Read the model definition and answer for the solid it produces. Units are mm, in the model's axes. A direction names the side the tool comes from. Coordinates: 2 decimals unless noted, no trailing zeros. Order: outer loops, then holes, each group sorted by start corner. A loop starts at its lowest first (then second) coordinate and runs counter-clockwise, first axis right, second up. Notation, with made-up numbers: (14, 23) -> (42, 23) arc R10 cw to (42, 32) -> close; hole circle Ø8 at (2, -0.5). An arc over 180 degrees is marked (long way). Answer as a JSON object with one key per item and string values. Group by question number.
1) Section D-D on z = 5.25 is taken. Determine the outline of the cut face in (x, y), and give its area (3 significant figures).
2) Section B-B on x = 86 is taken. Determine the outline of the cut face in (y, z), and give its area (3 significant figures).
3) Determine the mould class of faces 4 (the flat face through (13, 0, 0)), 5 (the cylindrical face through (128.719, -5.594, 10.26)), 6 (the cylindrical face through (119, 0, 10)), 7 (the cylindrical face through (4.8, -2.4, 0.7)) for opening direction X: released by +X, released by -X, zero draft, split by the parting line, or undercut.
4) Consider L1, parallel to Y at x = 8, z = 0.75; L2, parallel to Z at x = 15.5, y = 0.75; L3, parallel to Z at x = 49, y = -1.5. Determine where each line is inside the solid, lowest interval first.
5) A tool of negligible diameter and unlimited length cuts with its end or side. For faces 1 (the flat face through (82, 0, 9.5)), 2 (the flat face through (66, 8, 10)), 3 (the flat face through (13, 0, 1.5)), from which of +Z, -Z, +X, -X, +Y, -Y can it reach the whole face along a straight path? Write none if from no direction.
6) Given pin 1 (8 mm diameter, centred on x = 11.5, y = -0.5, fed in from +Z); pin 2 (5 mm diameter, centred on y = 2, z = 3, fed in from +X), each flat-ended and moving along its own axis, determine where each tip first touches the part or whether it passes through.
7) Section A-A on y = -1.25 is taken. Determine the outline of the cut face in (x, z).
8) Section C-C on y = -6.5 is taken. Determine the outline of the cut face in (x, z), and give its area (3 significant figures).
from build123d import *

# Parameters (mm, degrees)
EXTRUDE_1_DEPTH          = 8
FILLET_1_R               = 8
CUT_EXTRUDE_1_DEPTH      = 132.587423411
CUT_EXTRUDE_1_DEPTH_BACK = 132.587423411
SKETCH_2_R               = 4


with BuildPart() as part:
    # 草图1 → 拉伸-薄壁1 (new, symmetric)
    with BuildSketch(Plane(origin=(0, 0, 0), x_dir=(1, 0, 0), z_dir=(0, 1, 0))):
        Polygon((0, 0), (18, 0), (34, -9.5), (131, -9.5), (131, -11), (33.588243042, -11), (17.588243042, -1.5), (0, -1.5), align=None)
    extrude(amount=EXTRUDE_1_DEPTH, both=True)

    # 圆角1
    fillet_1_edges = [part.edges().sort_by_distance(p)[0] for p in [
        (131, -8, 10.25),
        (131, 8, 10.25),
        (0, -8, 0.75),
        (0, 8, 0.75),
    ]]
    fillet(fillet_1_edges, radius=FILLET_1_R - 0.0001)  # a hair under: the kernel refuses the full size

    # 草图2 → 切除-拉伸1 (cut, two sides: drawn at the far end of the back side and taken through both)
    with BuildSketch(Plane.XY.offset(1.5).offset(-CUT_EXTRUDE_1_DEPTH_BACK)):
        with Locations((8, 0)):
            Circle(SKETCH_2_R)
        with Locations((123, 0)):
            Circle(SKETCH_2_R)
    extrude(amount=CUT_EXTRUDE_1_DEPTH + CUT_EXTRUDE_1_DEPTH_BACK, mode=Mode.SUBTRACT)


solid = part.part
Worked answers:
{
 "1": {"outline": "(23.9, -8) -> (26.84, -8) -> (26.84, 8) -> (23.9, 8) -> close", "area": "47.0 mm²"},
 "2": {"outline": "(-8, 9.5) -> (8, 9.5) -> (8, 11) -> (-8, 11) -> close", "area": "24.0 mm²"},
 "3": {"face 4": "zero draft", "face 5": "released by +X", "face 6": "undercut", "face 7": "undercut"},
 "4": {"L1": "y = -8 to -4, 4 to 8", "L2": "z = 0 to 1.5", "L3": "z = 9.5 to 11"},
 "5": {"face 1": "-Z, +X, +Y, -Y", "face 2": "+Z, -Z, +X, -X, +Y", "face 3": "+Z, -X, +Y, -Y"},
 "6": {"pin 1": "stops at z = 1.5", "pin 2": "stops at x = 27.26"},
 "7": {"outline": "(0.1, 0) -> (4.2, 0) -> (4.2, 1.5) -> (0.1, 1.5) -> close; (11.8, 0) -> (18, 0) -> (34, 9.5) -> (119.2, 9.5) -> (119.2, 11) -> (33.59, 11) -> (17.59, 1.5) -> (11.8, 1.5) -> close; (126.8, 9.5) -> (130.9, 9.5) -> (130.9, 11) -> (126.8, 11) -> close"},
 "8": {"outline": "(3.34, 0) -> (18, 0) -> (34, 9.5) -> (127.66, 9.5) -> (127.66, 11) -> (33.59, 11) -> (17.59, 1.5) -> (3.34, 1.5) -> close", "area": "190 mm²"}
}
